```python
from build123d import *

# Parameters (mm, degrees)
ESQUISSE1_W                    = 85
ESQUISSE1_H                    = 55
BOSS_EXTRU_1_DEPTH             = 10
ESQUISSE2_W                    = 8
ESQUISSE2_H                    = 5
ESQUISSE2_W_2                  = 42
ENL_V_MAT_EXTRU_1_DEPTH        = 102.734949747
ESQUISSE3_R                    = 2
ENL_V_MAT_EXTRU_2_DEPTH        = 90.895772982
TROU_TARAUD_M3X0_51_AT_2_COUNT = 2
TROU_TARAUD_M3X0_51_AT_2_PITCH = 33
TROU_TARAUD_M3X0_51_AT_3_COUNT = 2
TROU_TARAUD_M3X0_51_AT_3_PITCH = 68
TROU_TARAUD_M3X0_52_D          = 2
TROU_TARAUD_M3X0_52_DEPTH      = 12
TROU_TARAUD_M3X0_52_TIP        = 0.600860619
ESQUISSE9_W                    = 6
ESQUISSE9_H                    = 30
ENL_V_MAT_EXTRU_4_DEPTH        = 90.895772982
CONG_1_R                       = 4


with BuildPart() as part:
    # Esquisse1 → Boss.-Extru.1 (new body)
    with BuildSketch(Plane.XY):
        with Locations((42.5, 0)):
            Rectangle(ESQUISSE1_W, ESQUISSE1_H)
    extrude(amount=BOSS_EXTRU_1_DEPTH)

    # Esquisse2 → Enlèv. mat.-Extru.1 (cut, through all)
    with BuildSketch(Plane(origin=(0, 27.5, 0), x_dir=(1, 0, 0), z_dir=(0, 1, 0))):
        with Locations((4, -2.5)):
            Rectangle(ESQUISSE2_W, ESQUISSE2_H)
        with Locations((54, -2.5)):
            Rectangle(ESQUISSE2_W_2, ESQUISSE2_H)
    extrude(amount=-ENL_V_MAT_EXTRU_1_DEPTH, mode=Mode.SUBTRACT)

    # Esquisse3 → Enlèv. mat.-Extru.2 (cut, through all)
    with BuildSketch(Plane.XY.offset(10)):
        with Locations((4, 0)):
            Circle(ESQUISSE3_R)
        with Locations((37, 0)):
            Circle(ESQUISSE3_R)
    extrude(amount=-ENL_V_MAT_EXTRU_2_DEPTH, mode=Mode.SUBTRACT)

    # Esquisse4 → Trou taraudé M3x0.51 (revolve, cut)
    with BuildSketch(Plane(origin=(4, -27.5, 7.5), x_dir=(0, 0, -1), z_dir=(1, 0, 0))):
        Polygon((0, 0), (0, 15.600860619), (1, 15), (1, 0), align=None)
    trou_taraud_m3x0_51 = revolve(axis=Axis((4, -33.85, 7.5), (0, 1, 0)), mode=Mode.SUBTRACT)

    # Trou taraudé M3x0.51 at 2: Trou taraudé M3x0.51 ×2
    with Locations(*[(i * TROU_TARAUD_M3X0_51_AT_2_PITCH, 0, 0) for i in range(1, TROU_TARAUD_M3X0_51_AT_2_COUNT)]):
        add(trou_taraud_m3x0_51, mode=Mode.SUBTRACT)

    # Trou taraudé M3x0.51 at 3: Trou taraudé M3x0.51 ×2
    with Locations(*[(i * TROU_TARAUD_M3X0_51_AT_3_PITCH, 0, 0) for i in range(1, TROU_TARAUD_M3X0_51_AT_3_COUNT)]):
        add(trou_taraud_m3x0_51, mode=Mode.SUBTRACT)

    # Symétrie1: Trou taraudé M3x0.51 across plane
    add(trou_taraud_m3x0_51.mirror(Plane.ZX), mode=Mode.SUBTRACT)

    # Symétrie1 copy 1 sketch → Symétrie1 copy 1 (revolve, cut)
    with BuildSketch(Plane(origin=(37, 27.5, 7.5), x_dir=(0, 0, -1), z_dir=(1, 0, 0))):
        Polygon((0, 0), (0, -15.600860619), (1, -15), (1, 0), align=None)
    revolve(axis=Axis((37, 33.85, 7.5), (0, 1, 0)), mode=Mode.SUBTRACT)

    # Symétrie1 copy 2 sketch → Symétrie1 copy 2 (revolve, cut)
    with BuildSketch(Plane(origin=(72, 27.5, 7.5), x_dir=(0, 0, -1), z_dir=(1, 0, 0))):
        Polygon((0, 0), (0, -15.600860619), (1, -15), (1, 0), align=None)
    revolve(axis=Axis((72, 33.85, 7.5), (0, 1, 0)), mode=Mode.SUBTRACT)

    # Trou taraudé M3x0.52
    with Locations(Plane(origin=(85, 0, 0), x_dir=(0, 0, -1), z_dir=(1, 0, 0))):
        with Locations((-5, 20), (-5, -20)):
            Hole(TROU_TARAUD_M3X0_52_D / 2, depth=TROU_TARAUD_M3X0_52_DEPTH)
            with Locations((0, 0, -(TROU_TARAUD_M3X0_52_DEPTH + TROU_TARAUD_M3X0_52_TIP / 2))):  # 118° drill point
                Cone(0, TROU_TARAUD_M3X0_52_D / 2, TROU_TARAUD_M3X0_52_TIP, mode=Mode.SUBTRACT)

    # Esquisse9 → Enlèv. mat.-Extru.4 (cut, through all)
    with BuildSketch(Plane.XY.offset(10)):
        with Locations((82, 0)):
            Rectangle(ESQUISSE9_W, ESQUISSE9_H)
    extrude(amount=-ENL_V_MAT_EXTRU_4_DEPTH, mode=Mode.SUBTRACT)

    # Congé1
    cong_1_edges = [part.edges().sort_by_distance(p)[0] for p in [
        (79, -15, 5),
        (79, 15, 5),
    ]]
    fillet(cong_1_edges, radius=CONG_1_R)


solid = part.part
```
Build history of the part. All positions in model axes, mm. A direction names the side the tool comes from. Round coordinates to 2 decimals unless told otherwise and drop trailing zeros. Write each loop counter-clockwise with the first axis right and the second up, starting at its lowest first coordinate (ties: lowest second). Pieces come first, ordered by that corner, then holes. Notation, with made-up numbers: (3, -20) - (8, -20) arc R18 cw to (8, 8) - close; hole circle Ø8 at (-15, 70). An arc over 180 degrees is marked (long way). Write each question's results on one line, items separated by ' | '. Start each with the question number.
Item 1: Which spindle directions (+Z, -Z, +X, -X, +Y, -Y) get a long thin tool onto all of the face, cutting with end or side? Do faces 1 (the face through (72.89, 20.1, 7.04)), 2 (the face through (8, 0, 3)), 3 (the face through (72.89, -20.1, 7.04)), 4 (the face through (33, 0, 3)), 5 (the face through (80.203, 13.859, 4.93)). Say none if no direction does.
Item 2: Saw through at D-D (y = 10). Write the cut outline in (x, z).
Item 3: Drop flat-ended pins along their axis: P1, Ø4.5, axis at x = 4, y = 0, coming from the -Z side; P2, Ø1.5, axis at y = 5, z = 2, coming from the -X side; P3, Ø4, axis at y = -6, z = 6.5, coming from the +X side. Give the stop position or say it passes through.
Item 4: Saw through at A-A (y = 20). Write the cut outline in (x, z).
Item 5: Saw through at B-B (z = 1). Write the cut outline in (x, y).
Item 6: Saw through at C-C (y = 0). Write the cut outline in (x, z).
Item 7: Wall check: L1, parallel to X at y = -23.5, z = 7.5; L2, parallel to Z at x = 37, y = -22; L3, parallel to Y at x = 81, z = 5. Give the ranges that are in metal, low to high. Write a range as [from, to].
Item 8: Mould opens along Y. For faces 6 (the face through (4.17, 12.003, 7.538)), 7 (the face through (0, 0, 7)), 8 (the face through (84, -15, 5)) say: pulls with the +Y half, pulls with the -Y half, needs draft (parallel to the pull), parting line crosses it, or undercut.
Results are:
1) face 1: +Y | face 2: -Z, -X, +Y, -Y | face 3: -Y | face 4: -Z, +Y, -Y | face 5: +Z, -Z, +X
2) outline: (0, 5) - (8, 5) - (8, 0) - (33, 0) - (33, 5) - (75, 5) - (75, 0) - (79, 0) - (79, 10) - (0, 10) - close
3) P1: stops at z = 5 | P2: stops at x = 8 | P3: stops at x = 79
4) outline: (0, 5) - (8, 5) - (8, 0) - (33, 0) - (33, 5) - (72.4, 5) - (73, 6) - (85, 6) - (85, 10) - (0, 10) - close; (75, 0) - (85, 0) - (85, 4) - (75, 4) - close; hole circle Ø2 at (4, 7.5); hole circle Ø2 at (37, 7.5); hole circle Ø2 at (72, 7.5)
5) outline: (8, -27.5) - (33, -27.5) - (33, 27.5) - (8, 27.5) - close; (75, -27.5) - (85, -27.5) - (85, -15) - (83, -15) arc R4 cw to (79, -11) - (79, 11) arc R4 cw to (83, 15) - (85, 15) - (85, 27.5) - (75, 27.5) - close
6) outline: (0, 5) - (2, 5) - (2, 10) - (0, 10) - close; (6, 5) - (8, 5) - (8, 0) - (33, 0) - (33, 5) - (35, 5) - (35, 10) - (6, 10) - close; (39, 5) - (75, 5) - (75, 0) - (79, 0) - (79, 10) - (39, 10) - close
7) L1: x = [0, 3], [5, 36], [38, 71], [73, 85] | L2: z = [5, 6.5], [8.5, 10] | L3: y = [-27.5, -21], [-19, -14.46], [14.46, 19], [21, 27.5]
8) face 6: pulls with the +Y half | face 7: needs draft | face 8: undercut
